Part model, mm, in its own coordinate system. Face numbers are marked on the shaded views. A direction names the side the tool comes from. Round coordinates to 2 decimals unless told otherwise and drop trailing zeros. Loops run counter-clockwise (first coordinate to the right, second up) from the corner with the lowest first, then second, coordinate; pieces in that order, holes last. Notation, with made-up numbers: (45.25, 0) -> (94.25, 0) arc R23 cw to (94.25, 14) -> close; hole circle Ø10 at (23, 74). An arc over 180 degrees is marked (long way). Use a Markdown table: item, result. Add a question column.
Item 1: Which spindle directions (+Z, -Z, +X, -X, +Y, -Y) get a long thin tool onto all of the face, cutting with end or side? Do the marked faces 1, 2, 3, 4 and 5. Say none if no direction does.
Item 2: Cut at B-B, the plane y = 2.75. List the corners of the cut face in (x, z).
Item 3: Probe line 1 (Y direction, x = -7.75, z = 1.5); line 2 (Z direction, x = -0.25, y = -11); line 3 (Y direction, x = -4.5, z = 2.15). List the from-to ranges inside material, lowest first. Write a range as [from, to].
Item 4: Two-plate mould, pull along Y, no slides. Class the marked faces 6, 7 and 8: pulls with the +Y half, pulls with the -Y half, needs draft (parallel to the pull), parting line crosses it, or undercut.
Item 5: Cut at C-C, the plane z = 0.25. List the corners of the cut face in (x, y), plus the area to 3 significant figures.
Item 6: Cut at A-A, the plane x = 7. List the corners of the cut face in (y, z), plus the area to 3 significant figures.
Item 7: Cut at D-D, the plane z = 1.1. List the corners of the cut face in (x, y).
Item 8: Flat gauge pins, fed straight in: pin 1 (0.7 mm diameter, centred on x = -7.5, z = 1.5, fed in from -Y); pin 2 (1.5 mm diameter, centred on y = 4.5, z = 1, fed in from -X); pin 3 (1.5 mm diameter, centred on y = -9.5, z = 2, fed in from -X); pin 4 (0.7 mm diameter, centred on x = -7, z = 1, fed in from +Y). Where does each tip first touch, or does it go through?
```python
from build123d import *

# Parameters (mm, degrees)
F0_W      = 17
F0_H      = 11
F1_DEPTH  = 3
F2_W      = 12
F2_H      = 3
F3_DEPTH  = 3.001
F4_W      = 1.5
F4_H      = 1.5
F5_DEPTH  = 100
F6_SIZE   = 1
F7_SIZE   = 1
F8_R      = 1
F9_DEPTH  = 3
F10_W     = 1.5
F10_H     = 3
F11_DEPTH = 3
F13_DEPTH = 9.251
F14_W     = 1.5
F14_H     = 1.416422517
F15_DEPTH = 25


with BuildPart() as f1:
    # F0 (on Top) → F1 (new body)
    with BuildSketch(Plane.XY):
        Rectangle(F0_W, F0_H)
    extrude(amount=F1_DEPTH)

    # F2 (on face) → F3 (cut, through all)
    with BuildSketch(Plane.XY.offset(3)):
        with Locations((0, 4)):
            Rectangle(F2_W, F2_H)
    extrude(amount=-F3_DEPTH, mode=Mode.SUBTRACT)

    # F4 (on face) → F5 (cut)
    with BuildSketch(Plane(origin=(6, 0, 0), x_dir=(0, -1, 0), z_dir=(-1, 0, 0))):
        with Locations((-4, 1.5)):
            Rectangle(F4_W, F4_H)
    extrude(amount=-F5_DEPTH, mode=Mode.SUBTRACT)

    # F6
    f6_edges = [f1.edges().sort_by_distance(p)[0] for p in [
        (-7.25, 5.5, 3),
        (7.25, 5.5, 3),
    ]]
    chamfer(f6_edges, length=F6_SIZE)

    # F7
    f7_edges = [f1.edges().sort_by_distance(p)[0] for p in [
        (-7.25, 5.5, 0),
        (7.25, 5.5, 0),
    ]]
    chamfer(f7_edges, length=F7_SIZE)

    # F8
    f8_edges = [f1.edges().sort_by_distance(p)[0] for p in [
        (-7.25, 5.5, 2),
        (7.25, 5.5, 2),
        (-7.25, 5.5, 1),
        (7.25, 5.5, 1),
    ]]
    fillet(f8_edges, radius=F8_R)

    # F9 (add): a face of the model
    f9_faces = [f1.faces().sort_by_distance(p)[0] for p in [
        (0, -5.5, 1.5),
    ]]
    extrude(f9_faces, amount=F9_DEPTH)

    # F10 (on face) → F11 (join)
    with BuildSketch(Plane.XZ.offset(8.5)):
        with Locations((0, 1.5)):
            Rectangle(F10_W, F10_H)
    extrude(amount=F11_DEPTH)

    # F12 (on face) → F13 (cut, through all)
    with BuildSketch(Plane.YZ.offset(0.75)):
        Polygon((-8.5, 3), (-11.5, 3), (-10.0618377328, 1.5503217001), align=None)
    extrude(amount=-F13_DEPTH, mode=Mode.SUBTRACT)

    # F14 (on face) → F15 (cut)
    with BuildSketch(Plane.YZ.offset(-6)):
        with Locations((4, 1.5)):
            Rectangle(F14_W, F14_H)
    extrude(amount=-F15_DEPTH, mode=Mode.SUBTRACT)


solid = f1.part
```
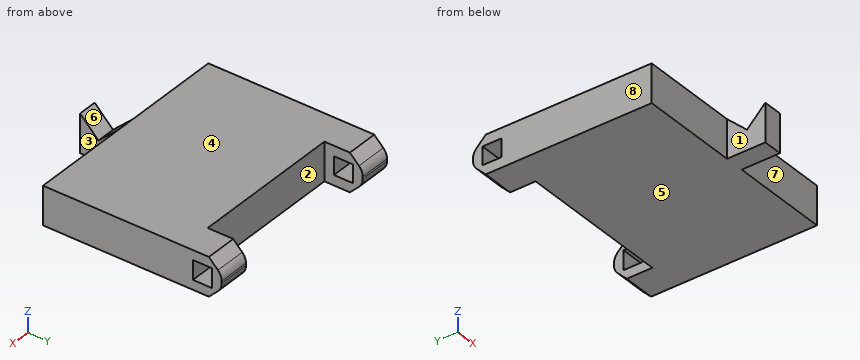
A:
| question | item | result |
|---|---|---|
| 1 | face 1 | +Z, -Z, -X, -Y |
| 1 | face 2 | +Z, -Z, +Y |
| 1 | face 3 | +Z, -Z, +X, -Y |
| 1 | face 4 | +Z, +X, -X, +Y, -Y |
| 1 | face 5 | -Z, +X, -X, +Y, -Y |
| 2 | outline | (-8.5, 0) -> (-6, 0) -> (-6, 3) -> (-8.5, 3) -> close; (6, 0) -> (8.5, 0) -> (8.5, 3) -> (6, 3) -> close |
| 3 | line 1 | y = [-8.5, 3.25], [4.75, 5.5] |
| 3 | line 2 | z = [0, 2.5] |
| 3 | line 3 | y = [-8.5, 2.5] |
| 4 | face 6 | undercut |
| 4 | face 7 | pulls with the -Y half |
| 4 | face 8 | needs draft |
| 5 | outline | (-8.5, -8.5) -> (-0.75, -8.5) -> (-0.75, -11.5) -> (0.75, -11.5) -> (0.75, -8.5) -> (8.5, -8.5) -> (8.5, 4.75) -> (6, 4.75) -> (6, 2.5) -> (-6, 2.5) -> (-6, 4.75) -> (-8.5, 4.75) -> close |
| 5 | area | 203 mm^2 |
| 6 | outline | (-8.5, 0) -> (4.5, 0) -> (5.21, 0.71) arc R1 ccw to (5.5, 1.41) -> (5.5, 1.59) arc R1 ccw to (5.21, 2.29) -> (4.5, 3) -> (-8.5, 3) -> close; hole (3.25, 0.75) -> (4.75, 0.75) -> (4.75, 2.25) -> (3.25, 2.25) -> close |
| 6 | area | 38.7 mm^2 |
| 7 | outline | (-8.5, -8.5) -> (-0.75, -8.5) -> (-0.75, -11.5) -> (0.75, -11.5) -> (0.75, -8.5) -> (8.5, -8.5) -> (8.5, 3.25) -> (6, 3.25) -> (6, 2.5) -> (-6, 2.5) -> (-6, 3.25) -> (-8.5, 3.25) -> close; (-8.5, 4.75) -> (-6, 4.75) -> (-6, 5.45) -> (-8.5, 5.45) -> close; (6, 4.75) -> (8.5, 4.75) -> (8.5, 5.45) -> (6, 5.45) -> close |
| 8 | pin 1 | stops at y = -8.5 |
| 8 | pin 2 | stops at x = -8.5 |
| 8 | pin 3 | stops at x = -0.75 |
| 8 | pin 4 | stops at y = 5.5 |
